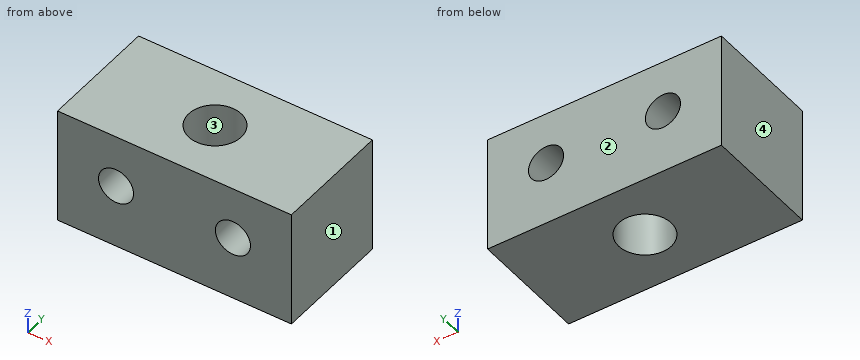
from build123d import *

# Parameters (mm, degrees)
ESQUISSE1_W                  = 20
ESQUISSE1_H                  = 10
BOSS_EXTRU_1_DEPTH           = 10
ESQUISSE2_R                  = 2.25
ENL_V_MAT_EXTRU_1_DEPTH      = 11
ESQUISSE3_R                  = 1.5
ENL_V_MAT_EXTRU_2_DEPTH      = 1
ENL_V_MAT_EXTRU_2_DEPTH_BACK = 11


with BuildPart() as part:
    # Esquisse1 → Boss.-Extru.1 (new body)
    with BuildSketch(Plane.XY):
        with Locations((10, 5)):
            Rectangle(ESQUISSE1_W, ESQUISSE1_H)
    extrude(amount=BOSS_EXTRU_1_DEPTH)

    # Esquisse2 → Enlèv. mat.-Extru.1 (cut, through all)
    with BuildSketch(Plane.XY.offset(10)):
        with Locations((10, 5)):
            Circle(ESQUISSE2_R)
    extrude(amount=-ENL_V_MAT_EXTRU_1_DEPTH, mode=Mode.SUBTRACT)

    # Esquisse3 → Enlèv. mat.-Extru.2 (cut, two sides)
    with BuildSketch(Plane(origin=(0, 10, 0), x_dir=(1, 0, 0), z_dir=(0, 1, 0))) as enl_v_mat_extru_2_sk:
        with Locations((5, -5.5)):
            Circle(ESQUISSE3_R)
        with Locations((15, -5.5)):
            Circle(ESQUISSE3_R)
    extrude(amount=ENL_V_MAT_EXTRU_2_DEPTH, mode=Mode.SUBTRACT)
    extrude(enl_v_mat_extru_2_sk.sketch, amount=-ENL_V_MAT_EXTRU_2_DEPTH_BACK, mode=Mode.SUBTRACT)


solid = part.part
Geometry: final body of the model. Coordinates: model frame, mm. Face numbers are marked on the shaded views. Give positions to 0.01 mm unless a question says otherwise; leave off trailing zeros. Loops run counter-clockwise (first coordinate to the right, second up) from the corner with the lowest first, then second, coordinate; pieces in that order, holes last. Notation, with made-up numbers: M -17,-23.75 L -9,-23.75 A22 cw -9,-12.75 Z; hole C 24.5,69 d2. An arc over 180 degrees is marked long. Put each result on its own line as item: value. Start each with the question number.
1) Cut plane D-D (x = 10). Output: boundary loops of the cut face in (y, z).
2) Cut plane B-B (y = 3). Output: boundary loops of the cut face in (x, z), then the cut area to 3 significant figures.
3) Ray query, line 1 along X through (y, z) = (7.75, 5.5); line 2 along Z through (x, y) = (5, 3); line 3 along Y through (x, z) = (10, 2). Return the intervals inside material, ascending.
4) Contact query for a flat-ended pin moving along its axis: pin 1 (1.5 mm diameter, centred on x = 7, z = 7, fed in from -Y). Output: stop coordinate, or through.
5) Cut plane A-A (x = 15). Output: boundary loops of the cut face in (y, z), then the cut area to 3 significant figures.
6) Pull-direction query (X, two-part tool) for the marked faces 1, 2, 3 and 4; classes: pulls with the +X half, pulls with the -X half, needs draft (parallel to the pull), parting line crosses it, or undercut.
7) Cut plane C-C (z = 4.5). Output: boundary loops of the cut face in (x, y).
Verdict:
1. outline: M 0,0 L 2.75,0 L 2.75,10 L 0,10 Z; M 7.25,0 L 10,0 L 10,10 L 7.25,10 Z
2. outline: M 0,0 L 8.97,0 L 8.97,10 L 0,10 Z; M 11.03,0 L 20,0 L 20,10 L 11.03,10 Z; hole C 5,5.5 d3; hole C 15,5.5 d3
2. area: 165 mm2
3. line 1: 0 to 3.5, 6.5 to 13.5, 16.5 to 20
3. line 2: 0 to 4, 7 to 10
3. line 3: 0 to 2.75, 7.25 to 10
4. pin 1: y = 0
5. outline: M 0,0 L 10,0 L 10,4 L 0,4 Z; M 0,7 L 10,7 L 10,10 L 0,10 Z
5. area: 70.0 mm2
6. face 1: pulls with the +X half
6. face 2: needs draft
6. face 3: undercut
6. face 4: pulls with the -X half
7. outline: M 0,0 L 3.88,0 L 3.88,10 L 0,10 Z; M 6.12,0 L 13.88,0 L 13.88,10 L 6.12,10 Z; M 16.12,0 L 20,0 L 20,10 L 16.12,10 Z; hole C 10,5 d4.5
